Drawing for the job (mm, zero at the part's lowest x, y, z). A direction names the side the tool comes from. Coordinates: 2 decimals unless noted, no trailing zeros. Write each loop counter-clockwise with the first axis right and the second up, starting at its lowest first coordinate (ties: lowest second). Pieces come first, ordered by that corner, then holes. Notation, with made-up numbers: (-27, 8.5) -> (9, 8.5) arc R17 cw to (9, 14.5) -> close; hole circle Ø10 at (27.5, -10.5). An arc over 180 degrees is marked (long way). Write item = value, one per line. Start each with the question number.
Q1. Pin check, flat tips, straight feed: P1, Ø7, axis at x = 34.5, z = 6.5, coming from the +Y side; P2, Ø1.5, axis at x = 44.5, y = 5, coming from the -Z side. Stop position of each tip, or through.
Q2. Band-saw the part on B-B, the plane z = 15. List the corners of the cut face in (x, y), plus the area to 3 significant figures.
Q3. Probe line 1 (X direction, y = 3.45, z = 28.8); line 2 (Z direction, x = 71, y = 2.5); line 3 (Z direction, x = 11, y = 1.3). List the from-to ranges inside material, lowest first.
Q4. Tool access for the marked faces 1, 2 and 3: list every direction of +Z, -Z, +X, -X, +Y, -Y with a clear straight run to the whole face (end or side of a thin tool).
Q5. Band-saw the part on C-C, the plane y = 5.2. List the corners of the cut face in (x, z), plus the area to 3 significant figures.
Q6. Pull direction X, two halves, no side cores. Call the marked faces 4, 5, 6 and 7: released by +X, released by -X, zero draft, split by the parting line, or undercut.
Q7. Band-saw the part on A-A, the plane x = 55. List the corners of the cut face in (y, z), plus the area to 3 significant figures.
Q8. Band-saw the part on D-D, the plane x = 38. List the corners of the cut face in (y, z).
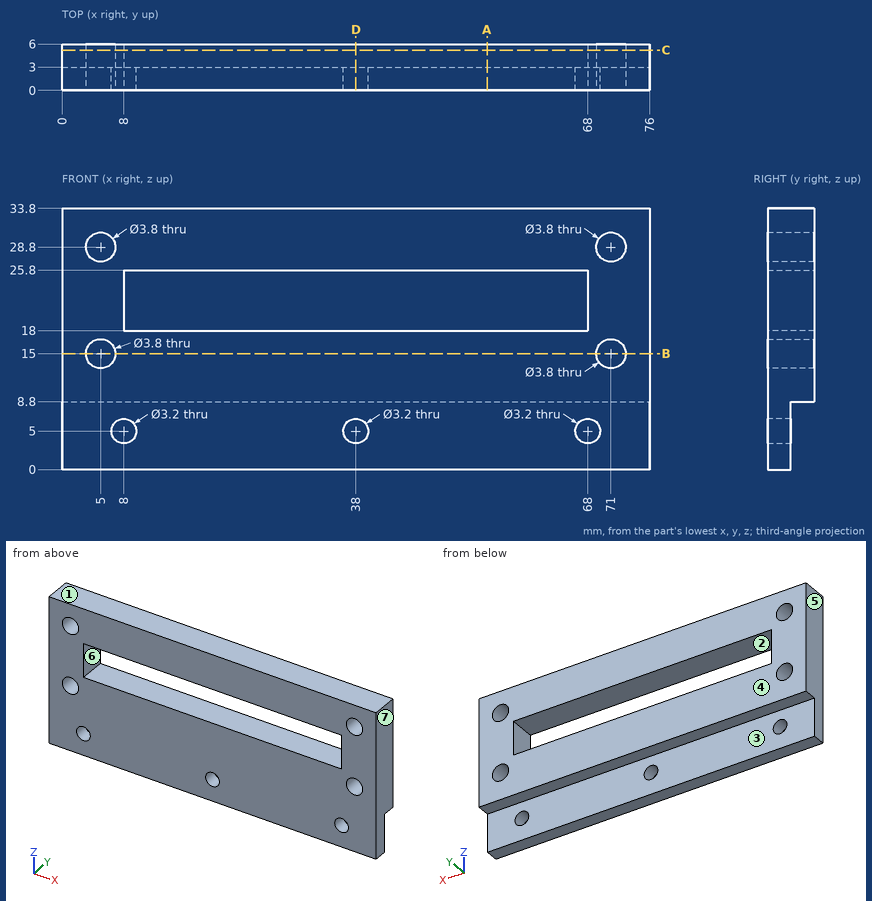
Ans:
q1.P1 = 6
q1.P2 = 8.8
q2.outline = (0, 0) -> (3.1, 0) -> (3.1, 6) -> (0, 6) -> close; (6.9, 0) -> (69.1, 0) -> (69.1, 6) -> (6.9, 6) -> close; (72.9, 0) -> (76, 0) -> (76, 6) -> (72.9, 6) -> close
q2.area = 410 mm2
q3.line_1 = 0 to 3.1, 6.9 to 69.1, 72.9 to 76
q3.line_2 = 0 to 13.1, 16.9 to 26.9, 30.7 to 33.8
q3.line_3 = 0 to 18, 25.8 to 33.8
q4.face_1 = +Z, +X, -X, +Y, -Y
q4.face_2 = +Y, -Y
q4.face_3 = -Z, +X, -X, +Y
q5.outline = (0, 8.8) -> (76, 8.8) -> (76, 33.8) -> (0, 33.8) -> close; hole circle Ø3.8 at (5, 15); hole circle Ø3.8 at (5, 28.8); hole (8, 18) -> (68, 18) -> (68, 25.8) -> (8, 25.8) -> close; hole circle Ø3.8 at (71, 15); hole circle Ø3.8 at (71, 28.8)
q5.area = 1,390 mm2
q6.face_4 = zero draft
q6.face_5 = released by -X
q6.face_6 = undercut
q6.face_7 = released by +X
q7.outline = (0, 0) -> (3, 0) -> (3, 8.8) -> (6, 8.8) -> (6, 18) -> (0, 18) -> close; (0, 25.8) -> (6, 25.8) -> (6, 33.8) -> (0, 33.8) -> close
q7.area = 130 mm2
q8.outline = (0, 0) -> (3, 0) -> (3, 3.4) -> (0, 3.4) -> close; (0, 6.6) -> (3, 6.6) -> (3, 8.8) -> (6, 8.8) -> (6, 18) -> (0, 18) -> close; (0, 25.8) -> (6, 25.8) -> (6, 33.8) -> (0, 33.8) -> close
